Design review of the part shown in the three views and the two pictorial views. Dimensions are in mm from the part's minimum x, y and z. Coordinates: 2 decimals unless noted, no trailing zeros. Write each loop counter-clockwise with the first axis right and the second up, starting at its lowest first coordinate (ties: lowest second). Pieces come first, ordered by that corner, then holes. Notation, with made-up numbers: (18, -35.5) -> (26, -35.5) arc R38 ccw to (26, 2.5) -> close; hole circle Ø2 at (-0.5, -25.5). An arc over 180 degrees is marked (long way). Write each question's results on one line, items separated by ' | '.
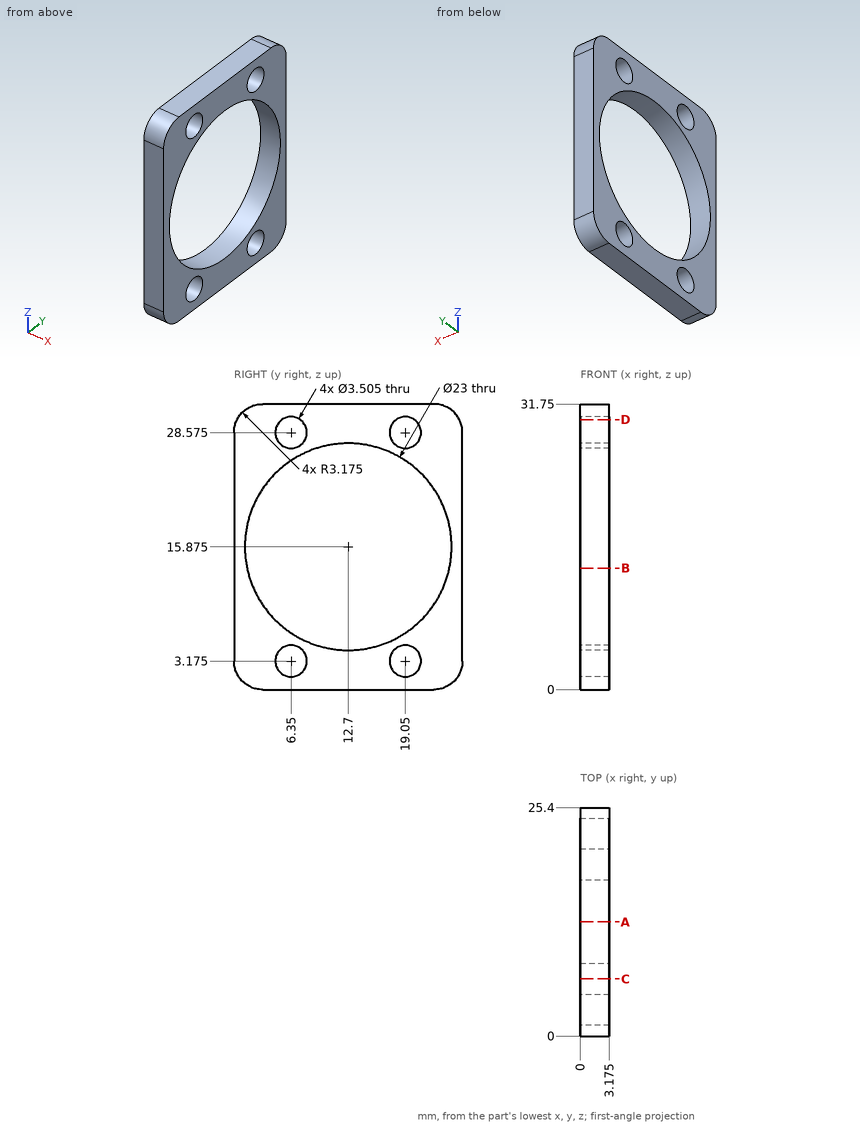
Q1. Clearance check with a flat-ended pin moving along its axis: P1, Ø2, axis at y = 6.35, z = 3.175, coming from the +X side. State where the tip first meets the part, or that it passes through.
Solution:
P1: through
Q2. Add section C-C (y = 6.35). Count the separate pieces of the cut face and the enclosed holes in it, plus the area to 3 significant figures.
Solution:
separate pieces: 4 | enclosed holes: 0 | area: 17.7 mm²
Q3. Add section B-B (z = 13.5). Write out the cut boundary in (x, y) (3 decimals).
Solution:
outline: (0, 0) -> (3.175, 0) -> (3.175, 1.448) -> (0, 1.448) -> close; (0, 23.952) -> (3.175, 23.952) -> (3.175, 25.4) -> (0, 25.4) -> close
Q4. For line 1 (Y direction, x = 2.8, z = 28.5); line 2 (Y direction, x = 0.1, z = 27.5) (1 decimal); line 3 (Z direction, x = 1.15, y = 19.05), list the stretches that pass through material, from the lowest coordinate up. Write a range as from..to.
Solution:
line 1: 0..4.6, 8.1..17.3, 20.8..25.4 | line 2: 0..5, 7.7..17.7, 20.4..25.4 | line 3: 0..1.42, 4.93..6.29, 25.46..26.82, 30.33..31.75
Q5. Add section A-A (y = 12.7). Write out the cut boundary in (x, z) (3 decimals), plus the area to 3 significant figures.
Solution:
outline: (0, 0) -> (3.175, 0) -> (3.175, 4.375) -> (0, 4.375) -> close; (0, 27.375) -> (3.175, 27.375) -> (3.175, 31.75) -> (0, 31.75) -> close | area: 27.8 mm²
Q6. Add section D-D (z = 30). Write out the cut boundary in (x, y) (1 decimal).
Solution:
outline: (0, 0.3) -> (3.2, 0.3) -> (3.2, 5.3) -> (0, 5.3) -> close; (0, 7.4) -> (3.2, 7.4) -> (3.2, 18) -> (0, 18) -> close; (0, 20.1) -> (3.2, 20.1) -> (3.2, 25.1) -> (0, 25.1) -> close
